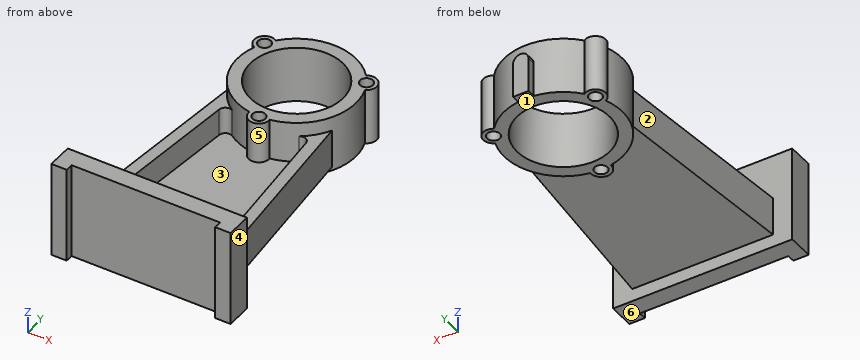
```python
from build123d import *

# Parameters (mm, degrees)
EXTRUDE_1_DEPTH             = 44
SKETCH_2_W                  = 75
SKETCH_2_H                  = 20
EXTRUDE_2_DEPTH             = 70
EXTRUDE_3_DEPTH             = 30
EXTRUDE_4_REACH             = 215.598
SKETCH_4_W                  = 9
SKETCH_4_H                  = 170
EXTRUDE_4_DIRECTION_2_REACH = 215.598
EXTRUDE_5_DEPTH             = 52
CUT_EXTRUDE_1_DEPTH         = 214.597752797
CUT_EXTRUDE_1_DEPTH_BACK    = 214.597752797
SKETCH_6_R                  = 36
SKETCH_6_R_2                = 5
SKETCH_6_W                  = 116
SKETCH_6_H                  = 6


with BuildPart() as part:
    # Sketch 1 → Extrude 1 (new body)
    with BuildSketch(Plane.XY):
        with BuildLine():
            ThreePointArc((7.969696861, -45.304347826), (39.837168574, -23), (43.21956455, 15.750213971))
            ThreePointArc((43.21956455, 15.750213971), (46.765371804, 27), (35.249867689, 29.554133855))
            ThreePointArc((35.249867689, 29.554133855), (0, 46), (-35.249867689, 29.554133855))
            ThreePointArc((-35.249867689, 29.554133855), (-46.765371804, 27), (-43.21956455, 15.750213971))
            ThreePointArc((-43.21956455, 15.750213971), (-39.837168574, -23), (-7.969696861, -45.304347826))
            ThreePointArc((-7.969696861, -45.304347826), (0, -54), (7.969696861, -45.304347826))
        make_face()
    extrude(amount=EXTRUDE_1_DEPTH)



with BuildPart() as body_2:
    # Sketch 2 → Extrude 2 (new, symmetric)
    with BuildSketch(Plane(origin=(0, 0, 0), x_dir=(0, 0, -1), z_dir=(1, 0, 0))):
        with Locations((-30.5, -180)):
            Rectangle(SKETCH_2_W, SKETCH_2_H)
    extrude(amount=EXTRUDE_2_DEPTH, both=True)


with BuildPart() as part_1:
    add(part.part)

    add(body_2.part)  # Extrude 3 merges body 2
    # Sketch 3 → Extrude 3 (add)
    with BuildSketch(Plane.XY.offset(3)):
        with BuildLine():
            Line((55, -170), (45.960435355, -170))
            Line((45.960435355, -170), (33.901757224, -41.537742182))
            ThreePointArc((33.901757224, -41.537742182), (31.040174213, -37.475102515), (26.087990263, -37.886894358))
            ThreePointArc((26.087990263, -37.886894358), (34.60790205, -30.303351559), (41, -20.856653615))
            Line((41, -20.856653615), (55, -170))
        make_face()
        with BuildLine():
            Line((-33.901757224, -41.537742182), (-45.960435355, -170))
            Line((-45.960435355, -170), (-55, -170))
            Line((-55, -170), (-41, -20.856653615))
            ThreePointArc((-41, -20.856653615), (-34.60790205, -30.303351559), (-26.087990263, -37.886894358))
            ThreePointArc((-26.087990263, -37.886894358), (-31.040174213, -37.475102515), (-33.901757224, -41.537742182))
        make_face()
    extrude(amount=EXTRUDE_3_DEPTH)

    # Sketch 4 → Extrude 4 (add, up to next)
    with BuildSketch(Plane(origin=(0, 0, 0), x_dir=(0, 0, -1), z_dir=(1, 0, 0)), mode=Mode.PRIVATE) as extrude_4_sk1:
        with Locations((-7.5, -85)):
            Rectangle(SKETCH_4_W, SKETCH_4_H)
    extrude_4_tool1 = extrude(extrude_4_sk1.sketch, amount=EXTRUDE_4_REACH, mode=Mode.PRIVATE) - part_1.part
    add(extrude_4_tool1.solids().sort_by_distance((0, -85, 7.5))[0])

    # Sketch 4 → Extrude 4 direction 2 (add, up to next)
    with BuildSketch(Plane(origin=(0, 0, 0), x_dir=(0, 0, -1), z_dir=(1, 0, 0)), mode=Mode.PRIVATE) as extrude_4_direction_2_sk1:
        with Locations((-7.5, -85)):
            Rectangle(SKETCH_4_W, SKETCH_4_H)
    extrude_4_direction_2_tool1 = extrude(extrude_4_direction_2_sk1.sketch, amount=-EXTRUDE_4_DIRECTION_2_REACH, mode=Mode.PRIVATE) - part_1.part
    add(extrude_4_direction_2_tool1.solids().sort_by_distance((0, -85, 7.5))[0])

    # Sketch 5 → Extrude 5 (add)
    with BuildSketch(Plane(origin=(0, 0, 0), x_dir=(1, 0, 0), z_dir=(0, 1, 0))):
        with BuildLine():
            Line((-6, -27), (-6, 0))
            Line((-6, 0), (6, 0))
            Line((6, 0), (6, -27))
            ThreePointArc((6, -27), (0, -33), (-6, -27))
        make_face()
    extrude(amount=EXTRUDE_5_DEPTH)

    # Sketch 6 → Cut-Extrude 1 (cut, two sides: drawn at the far end of the back side and taken through both)
    with BuildSketch(Plane.XY.offset(-CUT_EXTRUDE_1_DEPTH_BACK)):
        Circle(SKETCH_6_R)
        with Locations((0, -46)):
            Circle(SKETCH_6_R_2)
        with Locations((-39.837168574, 23)):
            Circle(SKETCH_6_R_2)
        with Locations((39.837168574, 23)):
            Circle(SKETCH_6_R_2)
        with Locations((0, -187)):
            Rectangle(SKETCH_6_W, SKETCH_6_H)
    extrude(amount=CUT_EXTRUDE_1_DEPTH + CUT_EXTRUDE_1_DEPTH_BACK, mode=Mode.SUBTRACT)


solid = part_1.part
```
Geometry check sheet. Reference: the model listing, model coordinates, mm. Face numbers are marked on the shaded views. A direction names the side the tool comes from. Coordinates: 2 decimals unless noted, no trailing zeros. Order: outer loops, then holes, each group sorted by start corner. A loop starts at its lowest first (then second) coordinate and runs counter-clockwise, first axis right, second up.
Q1. Draft check along X on the marked faces 4, 5 and 6. Enter one of: released by +X, released by -X, zero draft, split by the parting line, or undercut.
Reply:
face 4: released by +X
face 5: undercut
face 6: zero draft
Q2. Depth check by flat-ended pin: pin 1 Ø6 at (y, z) = (-113, 1.5) entering from +X; pin 2 Ø4 at (x, z) = (3, 57) entering from +Y; pin 3 Ø8 at (x, y) = (-39.84, 23) entering from -Z; pin 4 Ø6 at (x, z) = (-36.5, 23.5) entering from -Y. Enter the tip coordinate at first touch or a pass-through.
Reply:
pin 1: stops at x = 49.89
pin 2: stops at y = -170
pin 3: passes through
pin 4: stops at y = -184
Q3. Sectioned sample at A-A on x = 0. Record the cut outline in (y, z).
Reply:
outline: (-184, -7) - (-170, -7) - (-170, 3) - (-54, 3) - (-54, 0) - (-51, 0) - (-51, 44) - (-54, 44) - (-54, 12) - (-170, 12) - (-170, 68) - (-184, 68) - close; (-41, 0) - (-36, 0) - (-36, 44) - (-41, 44) - close; (36, 0) - (52, 0) - (52, 33) - (46, 33) - (46, 44) - (36, 44) - close
Q4. Sectioned sample at D-D on x = -16.5. Record the cut outline in (y, z), and give its area (3 significant figures).
Reply:
outline: (-184, -7) - (-170, -7) - (-170, 3) - (-42.94, 3) - (-42.94, 0) - (-32, 0) - (-32, 44) - (-42.94, 44) - (-42.94, 12) - (-170, 12) - (-170, 68) - (-184, 68) - close; (32, 0) - (42.94, 0) - (42.94, 44) - (32, 44) - close
area: 3,160 mm2
Q5. Tool access check on the marked faces 1, 2 and 3. Record the directions out of +Z, -Z, +X, -X, +Y, -Y that give a thin tool (end or side, any length) a straight path to the whole face; none if there is none.
Reply:
face 1: -Z, +X, -X, +Y
face 2: +Z, -Z, -X
face 3: +Z
Q6. Sectioned sample at B-B on z = 30. Give the number of separate pieces and of enclosed holes in the cut face, and give its area (3 significant figures).
Reply:
separate pieces: 1
enclosed holes: 5
area: 7,440 mm2
Q7. Thickness scan on probe 1 along Y at (x, z) = (0, 14); probe 2 along Y at (x, z) = (32.5, 25); probe 3 along X at (y, z) = (23, 33.5). Record the ranges inside material, lowest first.
Reply:
probe 1: y = -184 to -170, -54 to -51, -41 to -36, 36 to 52
probe 2: y = -184 to -170, -38.51 to -15.48, 15.48 to 32.55
probe 3: x = -47.84 to -44.84, -34.84 to -27.69, 27.69 to 34.84, 44.84 to 47.84
Q8. Sectioned sample at C-C on y = 23. Record the cut outline in (x, z).
Reply:
outline: (-47.84, 0) - (-44.84, 0) - (-44.84, 44) - (-47.84, 44) - close; (-34.84, 0) - (-27.69, 0) - (-27.69, 44) - (-34.84, 44) - close; (27.69, 0) - (34.84, 0) - (34.84, 44) - (27.69, 44) - close; (44.84, 0) - (47.84, 0) - (47.84, 44) - (44.84, 44) - close
